For this review, take the finished solid that the model builds, in its own axes (mm). A direction names the side the tool comes from. Round coordinates to 2 decimals unless told otherwise and drop trailing zeros. Order: outer loops, then holes, each group sorted by start corner. A loop starts at its lowest first (then second) coordinate and runs counter-clockwise, first axis right, second up. Notation, with made-up numbers: M 39,33 L 62,33 A30 cw 62,67 Z; hole C 42.5,-20.75 d11. An arc over 180 degrees is marked long. Answer as a JSON object with one key per item and string values.
from build123d import *

# Parameters (mm, degrees)
F0_W           = 9
F0_H           = 7.5
F0_W_2         = 13.5
F0_H_2         = 34.5
F1_DEPTH       = 39
F2_DEPTH       = 34
F3_D           = 2
F3_DEPTH       = 40
F3_START       = 34
F3_TIP         = 0.600860619
F4_DEPTH       = 3.5
F5_R           = 1.99999
F7_D           = 4
F7_DEPTH       = 10
F7_CBORE_D     = 9
F7_CBORE_DEPTH = 2.4
F7_TIP         = 1.2017212381
F8_DEPTH       = 50
F9_R           = 1


# Not quite as in the source:
# - a fillet or chamfer is up to 0.001 mm smaller than in the source, because OpenCascade refuses the exact size


with BuildPart() as f1:
    # F0 (on Front) → F1 (new body)
    with BuildSketch(Plane.XZ):
        Polygon((13.5, 0), (0, 0), (-13.5, 0), (-13.5, 34.5), (-13.5, 36), (-13.5, 46), (-17.5, 46), (-17.5, 0), (-17.5, -3), (-13.5, -3), (13.5, -3), align=None)
        Polygon((13.5, 34.5), (13.5, 0), (13.5, -3), (17.5, -3), (17.5, 0), (17.5, 46), (13.5, 46), align=None)
        Polygon((-13.5, 0), (0, 0), (0, 34.5), (-9, 34.5), (-13.5, 34.5), align=None)
        Polygon((0, 42), (0, 34.5), (13.5, 34.5), (13.5, 46), (-13.5, 46), (-13.5, 36), (-13.5, 34.5), (-9, 34.5), (-9, 42), align=None)
        with Locations((-4.5, 38.25)):
            Rectangle(F0_W, F0_H)
        with Locations((6.75, 17.25)):
            Rectangle(F0_W_2, F0_H_2)
    extrude(amount=-F1_DEPTH)

    # F0 (on Front) → F2 (cut)
    with BuildSketch(Plane.XZ):
        Polygon((-13.5, 0), (0, 0), (0, 34.5), (-9, 34.5), (-13.5, 34.5), align=None)
        with Locations((6.75, 17.25)):
            Rectangle(F0_W_2, F0_H_2)
        Polygon((0, 42), (0, 34.5), (13.5, 34.5), (13.5, 46), (-13.5, 46), (-13.5, 36), (-13.5, 34.5), (-9, 34.5), (-9, 42), align=None)
        with Locations((-4.5, 38.25)):
            Rectangle(F0_W, F0_H)
    extrude(amount=-F2_DEPTH, mode=Mode.SUBTRACT)

    # F3
    # its depths count from where the whole tool has entered the part; down to there all is cleared
    with Locations(Plane.XZ.offset(-F3_START)):
        with Locations((-9, 42), (9, 42)):
            Hole(F3_D / 2, depth=F3_DEPTH)
            with Locations((0, 0, -(F3_DEPTH + F3_TIP / 2))):  # 118° drill point
                Cone(0, F3_D / 2, F3_TIP, mode=Mode.SUBTRACT)

    # F0 (on Front) → F4 (join)
    with BuildSketch(Plane.XZ):
        Polygon((-13.5, 0), (0, 0), (0, 34.5), (-9, 34.5), (-13.5, 34.5), align=None)
        with Locations((6.75, 17.25)):
            Rectangle(F0_W_2, F0_H_2)
    extrude(amount=-F4_DEPTH)

    # F5 (radius 2 in the source; OpenCascade refuses exactly that, so slightly less here)
    f5_edges = [f1.edges().sort_by_distance(p)[0] for p in [
        (-15.5, 0, 46),
        (-17.5, 0, 21.5),
        (17.5, 0, 21.5),
        (15.5, 0, 46),
        (-17.5, 19.5, 46),
        (17.5, 19.5, 46),
        (0, 34, 46),
        (13.5, 17, 46),
        (-13.5, 17, 46),
        (0, 0, 34.5),
    ]]
    fillet(f5_edges, radius=F5_R)

    # F7
    with Locations(Plane.XZ.offset(-34)):
        with Locations((0, 36), (0, 16)):
            CounterBoreHole(F7_D / 2, F7_CBORE_D / 2, F7_CBORE_DEPTH, depth=F7_DEPTH)
            with Locations((0, 0, -(F7_DEPTH + F7_TIP / 2))):  # 118° drill point
                Cone(0, F7_D / 2, F7_TIP, mode=Mode.SUBTRACT)

    # F6 (on face) → F8 (cut)
    with BuildSketch(Plane.XZ.offset(-34)):
        with BuildLine():
            ThreePointArc((-5, 6.8252934143), (-3.5355339059, 3.2897595084), (0, 1.8252934143))
            Line((0, 1.8252934143), (0, 6.8252934143))
            Line((0, 6.8252934143), (-5, 6.8252934143))
        make_face()
        with BuildLine():
            Line((0, 6.8252934143), (0, 1.8252934143))
            ThreePointArc((0, 1.8252934143), (3.5355339059, 3.2897595084), (5, 6.8252934143))
            ThreePointArc((5, 6.8252934143), (3.5355339059, 10.3608273202), (0, 11.8252934143))
            Line((0, 11.8252934143), (0, 6.8252934143))
        make_face()
        with BuildLine():
            Line((-5, 6.8252934143), (0, 6.8252934143))
            Line((0, 6.8252934143), (0, 11.8252934143))
            ThreePointArc((0, 11.8252934143), (-3.5355339059, 10.3608273202), (-5, 6.8252934143))
        make_face()
        with BuildLine():
            Line((-5, 35.0794121623), (-5, 6.8252934143))
            ThreePointArc((-5, 6.8252934143), (-3.5355339059, 10.3608273202), (0, 11.8252934143))
            Line((0, 11.8252934143), (0, 16))
            Line((0, 16), (0, 35.0794121623))
            Line((0, 35.0794121623), (-5, 35.0794121623))
        make_face()
        with BuildLine():
            ThreePointArc((0, 11.8252934143), (3.5355339059, 10.3608273202), (5, 6.8252934143))
            Line((5, 6.8252934143), (5, 35.0794121623))
            Line((5, 35.0794121623), (0, 35.0794121623))
            Line((0, 35.0794121623), (0, 16))
            Line((0, 16), (0, 11.8252934143))
        make_face()
    extrude(amount=F8_DEPTH, mode=Mode.SUBTRACT)

    # F9
    f9_edges = [f1.edges().sort_by_distance(p)[0] for p in [
        (5, 3.5, 20.662647),
        (5, 0, 19.662652),
        (0, 3.5, 1.825293),
    ]]
    fillet(f9_edges, radius=F9_R)


solid = f1.part
1) Mouldability with a two-part tool opening along X and no side actions: class faces 1 (the cylindrical face through (16.9, 20.76, 45.43)), 2 (the cylindrical face through (-9, 37, 43)), 3 (the flat face through (-10, 3, 34.5)), 4 (the flat face through (0, 38, 46)) as +X half, -X half, draft (parallel to the pull), parting line (faces both ways), or undercut.
Geometry check:
{"face 1": "+X half", "face 2": "undercut", "face 3": "undercut", "face 4": "draft"}
2) Add section B-B on z = 36. State the section outline as (x, y) points, and give its area (3 significant figures).
Geometry check:
{"outline": "M -17.5,2 A2 ccw -15.5,0 L -13.5,0 L -13.5,34 L -4.5,34 L -4.5,36.4 L -2,36.4 L -2,39 L -17.5,39 Z; M 2,36.4 L 4.5,36.4 L 4.5,34 L 13.5,34 L 13.5,0 L 15.5,0 A2 ccw 17.5,2 L 17.5,39 L 2,39 Z", "area": "413 mm²"}
3) Add section A-A on z = 42. State the section outline as (x, y) points, and give its area (3 significant figures).
Geometry check:
{"outline": "M -17.5,2 A2 ccw -15.5,0 L -13.5,0 L -13.5,34 L -10,34 L -10,39 L -17.5,39 Z; M -8,34 L 8,34 L 8,39 L -8,39 Z; M 10,34 L 13.5,34 L 13.5,0 L 15.5,0 A2 ccw 17.5,2 L 17.5,39 L 10,39 Z", "area": "425 mm²"}
4) Add section D-D on z = 16. State the section outline as (x, y) points.
Geometry check:
{"outline": "M -17.5,2 A2 ccw -15.5,0 L -6,0 A1 ccw -5,1 L -5,2.5 A1 ccw -6,3.5 L -13.5,3.5 L -13.5,34 L -4.5,34 L -4.5,36.4 L -2,36.4 L -2,39 L -17.5,39 Z; M 2,36.4 L 4.5,36.4 L 4.5,34 L 13.5,34 L 13.5,3.5 L 6,3.5 A1 ccw 5,2.5 L 5,1 A1 ccw 6,0 L 15.5,0 A2 ccw 17.5,2 L 17.5,39 L 2,39 Z"}
5) For L1, parallel to X at y = 9, z = 23; L2, parallel to Z at x = 0, y = 37; L3, parallel to Y at x = 8.5, z = 28, list the stretches that pass through material, from the lowest coordinate up.
Geometry check:
{"L1": "x = -17.5 to -13.5, 13.5 to 17.5", "L2": "z = -3 to 14, 18 to 34, 38 to 46", "L3": "y = 0 to 3.5, 34 to 39"}
6) Machinability: for faces 5 (the flat face through (13.5, 17, 22)), 6 (the cylindrical face through (-0.22, 34.6, 45.43)), 7 (the cylindrical face through (-16.9, 0.57, 20.17)), 8 (the cylindrical face through (-0.98, 35.18, 31.61)), which of the approach directions +Z, -Z, +X, -X, +Y, -Y give a long, thin tool a straight path to every point of the face, cutting with its end or side? Answer none if there is none.
Geometry check:
{"face 5": "+Z", "face 6": "+Z, -Y", "face 7": "+Z, -Z, -X, -Y", "face 8": "-Y"}
7) Insertion check: P1, Ø1.5, axis at x = 8.5, y = 28, coming from the +Z side; P2, Ø4.5, axis at x = -0.5, z = 18, coming from the -Y side; P3, Ø1.2, axis at x = -9, z = 42, coming from the +Y side; P4, Ø2, axis at x = 4.5, z = 12, coming from the -Y side. Each pin has a flat end and moves straight along its axis. Give the tip position at first contact, or say it passes through.
Geometry check:
{"P1": "stops at z = 0", "P2": "stops at y = 36.4", "P3": "passes through", "P4": "stops at y = 0.13"}
